Here's the drawing with two shaded views (mm, measured from the low corner). I have some questions. Round coordinates to 2 decimals unless told otherwise and drop trailing zeros. Write each loop counter-clockwise with the first axis right and the second up, starting at its lowest first coordinate (ties: lowest second). Pieces come first, ordered by that corner, then holes. Notation, with made-up numbers: M 28,20.5 L 35,20.5 A37 cw 35,57.5 Z; hole C -39.75,71.5 d9. An arc over 180 degrees is marked long. Answer as a JSON object with one key per item and string values. Group by question number.
1) Suppose I cut it at C-C, the plane z = 27. Write out the boundary of the cut face in (x, y) (1 decimal), and give its area (3 significant figures).
2) Suppose I cut it at D-D, the plane y = 120. Write out the boundary of the cut face in (x, z).
3) Suppose I cut it at B-B, the plane x = 16.5. Write out the boundary of the cut face in (y, z), and give its area (3 significant figures).
4) I'm going to push flat-ended pins straight in: pin 1 Ø4 at (x, y) = (3.5, 77.5) entering from -Z; pin 2 Ø3 at (y, z) = (118, 17.5) entering from -X; pin 3 Ø2 at (x, y) = (12.5, 101) entering from -Z. Where does each tip first touch, or does it pass through?
5) Suppose I cut it at A-A, the plane z = 15.24. Write out the boundary of the cut face in (x, y), and give its area (3 significant figures).
6) Please list where these lines run through material, in increasing order: L1, parallel to Y at x = 7.25, z = 25.5; L2, parallel to X at y = 101.5, z = 15.5 (1 decimal); L3, parallel to Z at x = 6, y = 56. Write a range as [from, to].
7) If we mould it in two halves opening along Y, with no side actions, what happens to the marked faces 1, 2 and 3? For each: +Y half, -Y half, draft (parallel to the pull), parting line (faces both ways), or undercut.
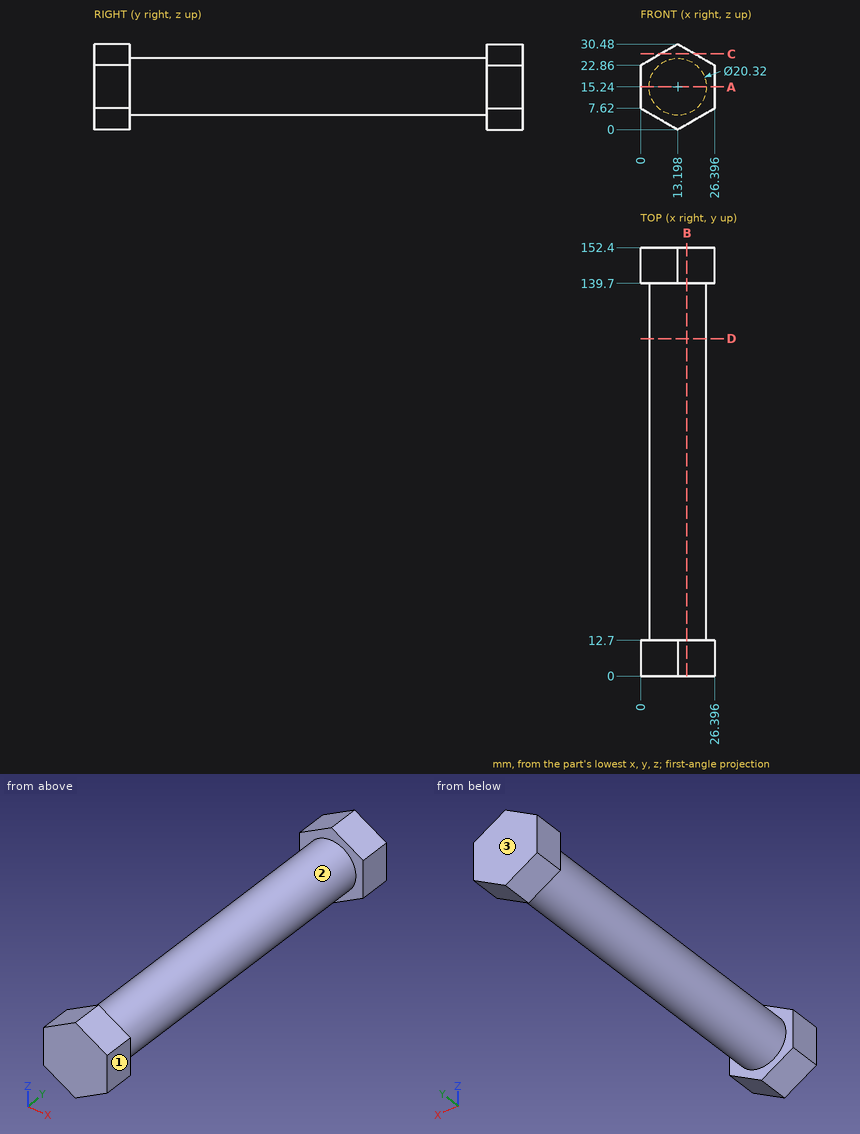
Results:
{
 "1": {"outline": "M 7.2,0 L 19.2,0 L 19.2,12.7 L 7.2,12.7 Z; M 7.2,139.7 L 19.2,139.7 L 19.2,152.4 L 7.2,152.4 Z", "area": "306 mm^2"},
 "2": {"outline": "C 13.2,15.24 d20.32"},
 "3": {"outline": "M 0,1.91 L 12.7,1.91 L 12.7,5.63 L 139.7,5.63 L 139.7,1.91 L 152.4,1.91 L 152.4,28.57 L 139.7,28.57 L 139.7,24.85 L 12.7,24.85 L 12.7,28.57 L 0,28.57 Z", "area": "3,120 mm^2"},
 "4": {"pin 1": "z = 8.61", "pin 2": "x = 3.07", "pin 3": "z = 5.08"},
 "5": {"outline": "M 0,0 L 26.4,0 L 26.4,12.7 L 23.36,12.7 L 23.36,139.7 L 26.4,139.7 L 26.4,152.4 L 0,152.4 L 0,139.7 L 3.04,139.7 L 3.04,12.7 L 0,12.7 Z", "area": "3,250 mm^2"},
 "6": {"L1": "[0, 12.7], [139.7, 152.4]", "L2": "[3, 23.4]", "L3": "[8.07, 22.41]"},
 "7": {"face 1": "draft", "face 2": "undercut", "face 3": "+Y half"}
}
